from build123d import *

# Parameters (mm, degrees)
SALIENTE_EXTRUIR1_DEPTH = 12.6
CROQUIS2_R              = 1
CROQUIS2_W              = 0.933974596
CROQUIS2_H              = 1
CORTAR_EXTRUIR2_DEPTH   = 2.5
CROQUIS4_R              = 6.3
CROQUIS4_R_2            = 2.5
CROQUIS4_R_3            = 2.4
CROQUIS4_W              = 4.8
CROQUIS4_H              = 4.8
SALIENTE_EXTRUIR4_DEPTH = 4.4


with BuildPart() as part:
    # Croquis1 → Saliente-Extruir1 (new body)
    with BuildSketch(Plane.XY):
        Polygon((11.5, 0), (-11.5, 0), (-11.5, 15.9), (-16.3, 15.9), (-16.3, 18.4), (-11.5, 18.4), (-11.5, 22.6), (11.5, 22.6), (11.5, 18.4), (16.3, 18.4), (16.3, 15.9), (11.5, 15.9), align=None)
    extrude(amount=SALIENTE_EXTRUIR1_DEPTH)

    # Croquis2 → Cortar-Extruir2 (cut)
    with BuildSketch(Plane(origin=(0, 18.4, 0), x_dir=(1, 0, 0), z_dir=(0, 1, 0))):
        with Locations((-14.5, -6.3)):
            Circle(CROQUIS2_R)
        with Locations((14.5, -6.3)):
            Circle(CROQUIS2_R)
        with Locations((-15.833012702, -6.3)):
            Rectangle(CROQUIS2_W, CROQUIS2_H)
        with Locations((15.833012702, -6.3)):
            Rectangle(CROQUIS2_W, CROQUIS2_H)
    extrude(amount=-CORTAR_EXTRUIR2_DEPTH, mode=Mode.SUBTRACT)

    # Croquis4 → Saliente-Extruir4 (add)
    with BuildSketch(Plane(origin=(0, 22.6, 0), x_dir=(1, 0, 0), z_dir=(0, 1, 0))):
        with Locations((-5.2, -6.3)):
            Circle(CROQUIS4_R)
        with Locations((-5.2, -6.3)):
            Circle(CROQUIS4_R_2, mode=Mode.SUBTRACT)
        with Locations((3.5, -6.3)):
            Circle(CROQUIS4_R_3)
        with Locations((1.1, -6.3)):
            Rectangle(CROQUIS4_W, CROQUIS4_H)
    extrude(amount=SALIENTE_EXTRUIR4_DEPTH)


solid = part.part
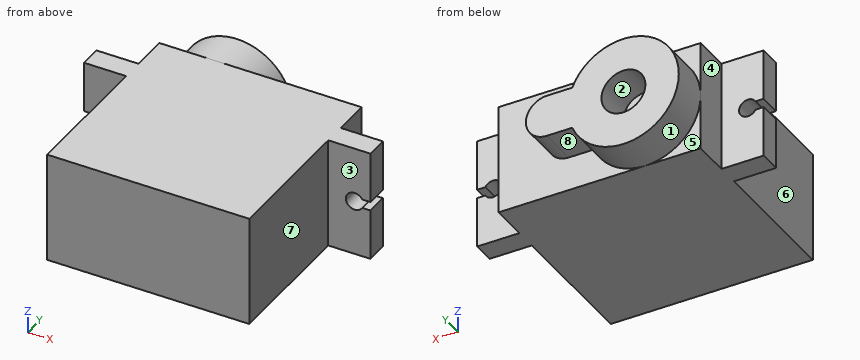
Source: CAD feature listing. Evaluate the final solid. Frame: model axes, mm. Face numbers are marked on the shaded views. A direction names the side the tool comes from. Give positions to 0.01 mm unless a question says otherwise; leave off trailing zeros. Write each loop counter-clockwise with the first axis right and the second up, starting at its lowest first coordinate (ties: lowest second). Pieces come first, ordered by that corner, then holes. Notation, with made-up numbers: (3, 25) -> (44, 25) arc R19 ccw to (44, 59) -> close; hole circle Ø1 at (0, 80.5). An arc over 180 degrees is marked (long way). Write item = value, one per line.
Q1. Line query: line 1 (X direction, y = 25.1, z = 6.3); line 2 (Z direction, x = -14.5, y = 17.55); line 3 (Y direction, x = 9.5, z = 7). Output: solid intervals per line, ascending. Write a range as from..to.
Here are the results:
line_1 = -11.5..-7.7, -2.7..5.9
line_2 = 0..5.3, 7.3..12.6
line_3 = 0..22.6
Q2. First-contact query: pin 1 (1.3 mm diameter, centred on y = 20, z = 6, fed in from +X); pin 2 (1 mm diameter, centred on y = 22.5, z = 7.5, fed in from -X); pin 3 (4 mm diameter, centred on x = 14.5, z = 4.5, fed in from +Y); pin 4 (1.2 mm diameter, centred on x = -14.5, z = 6.3, fed in from -Y). Flat tips, straight axial feed; report the tip coordinate or a pass-through.
Here are the results:
pin_1 = 11.5
pin_2 = -11.5
pin_3 = 18.4
pin_4 = through
Q3. Cut plane C-C on z = 2. Return loops of the section in (x, y).
Here are the results:
outline = (-16.3, 15.9) -> (-11.5, 15.9) -> (-11.5, 0) -> (11.5, 0) -> (11.5, 15.9) -> (16.3, 15.9) -> (16.3, 18.4) -> (11.5, 18.4) -> (11.5, 22.6) -> (-0.6, 22.6) -> (-0.6, 27) -> (-9.8, 27) -> (-9.8, 22.6) -> (-11.5, 22.6) -> (-11.5, 18.4) -> (-16.3, 18.4) -> close
Q4. Cut plane D-D on y = 11.5. Return loops of the section in (x, z), then the cut area to 3 significant figures.
Here are the results:
outline = (-11.5, 0) -> (11.5, 0) -> (11.5, 12.6) -> (-11.5, 12.6) -> close
area = 290 mm²
Q5. Reachability of the marked faces 4, 5, 6, 7 and 8 from +Z, -Z, +X, -X, +Y, -Y: full face, straight path, thin tool, end or side. Return the list, or none.
Here are the results:
face_4 = +Z, -Z, -X, +Y
face_5 = -Z, -X, +Y
face_6 = +Z, -Z, -X, -Y
face_7 = +Z, -Z, +X, -Y
face_8 = -Z, +X, +Y
Q6. Cut plane A-A on x = 14.5. Return loops of the section in (y, z), then the cut area to 3 significant figures.
Here are the results:
outline = (15.9, 0) -> (18.4, 0) -> (18.4, 5.3) -> (15.9, 5.3) -> close; (15.9, 7.3) -> (18.4, 7.3) -> (18.4, 12.6) -> (15.9, 12.6) -> close
area = 26.5 mm²
Q7. Mould query, pull axis X, two halves, no side actions, for the marked faces 1, 2 and 3. Classes: +X half, -X half, draft (parallel to the pull), parting line (faces both ways), or undercut.
Here are the results:
face_1 = parting line
face_2 = undercut
face_3 = draft
Q8. Cut plane B-B on x = 2.5. Return loops of the section in (y, z), then the cut area to 3 significant figures.
Here are the results:
outline = (0, 0) -> (22.6, 0) -> (22.6, 3.9) -> (27, 3.9) -> (27, 8.7) -> (22.6, 8.7) -> (22.6, 12.6) -> (0, 12.6) -> close
area = 306 mm²
